from build123d import *

# Parameters (mm, degrees)
SKETCH1_R           = 3.96875
BOSS_EXTRUDE1_DEPTH = 380
CHAMFER2_SIZE       = 1
CHAMFER3_SIZE       = 1


with BuildPart() as part:
    # Sketch1 → Boss-Extrude1 (new body)
    with BuildSketch(Plane.XY):
        Circle(SKETCH1_R)
    extrude(amount=BOSS_EXTRUDE1_DEPTH)

    # Chamfer2
    chamfer2_edges = [part.edges().sort_by_distance(p)[0] for p in [
        (-3.96875, 0, 0),
    ]]
    chamfer(chamfer2_edges, length=CHAMFER2_SIZE)

    # Chamfer3
    chamfer3_edges = [part.edges().sort_by_distance(p)[0] for p in [
        (-3.96875, 0, 380),
    ]]
    chamfer(chamfer3_edges, length=CHAMFER3_SIZE)


solid = part.part
Design review of the part built by this model. Coordinates are the model's own, in mm. Coordinates: 2 decimals unless noted, no trailing zeros. Loops run counter-clockwise (first coordinate to the right, second up) from the corner with the lowest first, then second, coordinate; pieces in that order, holes last. Notation, with made-up numbers: M 42,46 L 57,46 A24 cw 57,81 Z; hole C 34,56 d4. An arc over 180 degrees is marked long. Answer as CSV lines item,"result".
Item 1: For probe 1 along X at (y, z) = (0.5, 349); probe 2 along Y at (x, z) = (-0.75, 245); probe 3 along Y at (x, z) = (3, 31.5), list the stretches that pass through material, from the lowest coordinate up.
Answer list:
probe 1,"-3.94 to 3.94"
probe 2,"-3.9 to 3.9"
probe 3,"-2.6 to 2.6"
Item 2: Add section A-A on z = 131.5. State the section outline as (x, y) points, plus the area to 3 significant figures.
Answer list:
outline,"C 0,0 d7.94"
area,"49.5 mm²"
Item 3: For P1, Ø3, axis at y = 2.5, z = 175, coming from the -X side, flat-tipped, find the tip position at first contact; note if it passes through.
Answer list:
P1,"x = -3.84"
